Read the model definition and answer for the solid it produces. Units are mm, in the model's axes. A direction names the side the tool comes from. Coordinates: 2 decimals unless noted, no trailing zeros. Write each loop counter-clockwise with the first axis right and the second up, starting at its lowest first coordinate (ties: lowest second). Pieces come first, ordered by that corner, then holes. Notation, with made-up numbers: (-10.75, 83) -> (-6.75, 83) arc R29 cw to (-6.75, 111) -> close; hole circle Ø6 at (-0.75, 34). An arc over 180 degrees is marked (long way). Write item = value, one per line. Start each with the question number.
1) A flat-ended cylindrical pin translates along its axis: pin 1 Ø1 at (x, y) = (18.5, 42) entering from +Z. Find the tip coordinate at first contact, or state that the pin passes through.
2) Section C-C (y = 54) is taken. Determine the outline of the cut face in (x, z).
3) For a pull along Z with two mould halves and no side action, classify faces 1 (the face through (18, 33, -26.518)), 2 (the face through (18.44, -43.57, -17.24)), 3 (the face through (18.44, 65.82, -0.74)), 4 (the face through (20.002, -7, -20)) as released by +Z, released by -Z, zero draft, split by the parting line, or undercut.
4) A tool of negligible diameter and unlimited length cuts with its end or side. For faces 5 (the face through (18.437, 77.754, -8.06)), 6 (the face through (18, 1, -3.353)), from which of +Z, -Z, +X, -X, +Y, -Y can it reach the whole face along a straight path? Write none if from no direction.
5) Section A-A (y = -36) is taken. Determine the outline of the cut face in (x, z), plus the area to 3 significant figures.
6) Section D-D (z = -41.5) is taken. Determine the outline of the cut face in (x, y), plus the area to 3 significant figures.
7) Section B-B (x = 18.1) is taken. Determine the outline of the cut face in (y, z).
8) Find the intervals of material crossed by line 1 along Z through (x, y) = (18, 4.5); line 2 along Y through (x, z) = (18.45, -29); line 3 along Y through (x, z) = (19, -33), in increasing order. Write a range as from..to.
Solid Edge part; units mm, degrees
sketch "Sketch1" plane through (20.0025, 0, 0) normal (1, 0, 0) x (0, 1, 0)
  line L0 (82.357, -16.0334) -> (64.1977, -26.5176)
  line L1 (64.1977, -26.5176) -> (1.2767, -26.5176)
  line L2 (1.2767, -26.5176) -> (-52.04, -55.3528)
  line L3 (-52.04, -55.3528) -> (-62.8528, -55.3528)
  line L4 (-62.8528, -6.7056) -> (-62.8528, -55.3528)
  line L5 (-59.5, -3.3528) -> (-62.8528, -6.7056)
  line L6 (59.5, -3.3528) -> (-59.5, -3.3528)
  arc A0 (59.5, -3.3528) -> (62.8528, -2.4544) centre (59.5, 3.3528) ccw
  line L7 (68.6974, 0.92) -> (62.8528, -2.4544)
  arc A1 (73.2775, -0.3072) -> (68.6974, 0.92) centre (70.3738, -1.9836) ccw
  line L8 (73.2775, -0.3072) -> (82.357, -16.0334)
  circle A2 centre (-36.2028, -24.0028) radius 10
extrude "ExtrudedProtrusion_1" add sketch "Sketch1" against normal blind 3.175
properties material "Steel"
Answer key:
q1.pin_1 = -3.35
q2.outline = (16.83, -26.52) -> (20, -26.52) -> (20, -3.35) -> (16.83, -3.35) -> close
q3.face_1 = released by -Z
q3.face_2 = undercut
q3.face_3 = released by +Z
q3.face_4 = zero draft
q4.face_5 = +Z, +X, -X, +Y
q4.face_6 = +Z, +X, -X, -Y
q5.outline = (16.83, -46.68) -> (20, -46.68) -> (20, -34) -> (16.83, -34) -> close; (16.83, -14) -> (20, -14) -> (20, -3.35) -> (16.83, -3.35) -> close
q5.area = 74.1 mm^2
q6.outline = (16.83, -62.85) -> (20, -62.85) -> (20, -26.43) -> (16.83, -26.43) -> close
q6.area = 116 mm^2
q7.outline = (-62.85, -55.35) -> (-52.04, -55.35) -> (1.28, -26.52) -> (64.2, -26.52) -> (82.36, -16.03) -> (73.28, -0.31) arc R3.35 ccw to (68.7, 0.92) -> (62.85, -2.45) arc R6.71 cw to (59.5, -3.35) -> (-59.5, -3.35) -> (-62.85, -6.71) -> close; hole circle Ø20 at (-36.2, -24)
q8.line_1 = -26.52..-3.35
q8.line_2 = -62.85..-44.86, -27.54..-3.31
q8.line_3 = -62.85..-40.57, -31.84..-10.71
